Verification items for this drawing (mm, ordinates from the low corner). A direction names the side the tool comes from. Round coordinates to 2 decimals unless told otherwise and drop trailing zeros. Order: outer loops, then holes, each group sorted by start corner. A loop starts at its lowest first (then second) coordinate and runs counter-clockwise, first axis right, second up. Notation, with made-up numbers: (61, 87) -> (116, 87) arc R11 ccw to (116, 107) -> close; hole circle Ø5 at (88.5, 22.25). An arc over 180 degrees is marked (long way). Return JSON: item names as keys, results as strings. Group by question number.
Item 1: Sectioned sample at B-B on x = 114.3. Record the cut outline in (y, z).
Item 2: Access from +Z, -Z, +X, -X, +Y, -Y to the whole of each face (thin tool, end or side, straight path). Record for the marked faces 1, 2, 3, 4 and 5.
Item 3: Scan lines: probe 1 along Z at (x, y) = (31, 31.5); probe 2 along X at (y, z) = (19.05, 36); probe 3 along Y at (x, z) = (114.3, 28). Record each from-to range of solid material in increasing order. Write a range as from..to.
Item 4: Depth check by flat-ended pin: pin 1 Ø2 at (y, z) = (10.5, 32) entering from -X; pin 2 Ø6 at (y, z) = (29.5, 14) entering from -X; pin 3 Ø14.5 at (x, y) = (12.7, 19.05) entering from -Z; pin 4 Ø6 at (x, z) = (57, 23) entering from -Y. Enter the tip coordinate at first touch or a pass-through.
Item 5: Sectioned sample at A-A on z = 27. Record the cut outline in (x, y) (3 decimals), plus the area to 3 significant figures.
Item 6: Sectioned sample at D-D on x = 15.5. Record the cut outline in (y, z), plus the area to 3 significant figures.
Item 7: Sectioned sample at C-C on y = 10.5. Give the number of separate pieces and of enclosed holes in the cut face, plus the area to 3 significant figures.
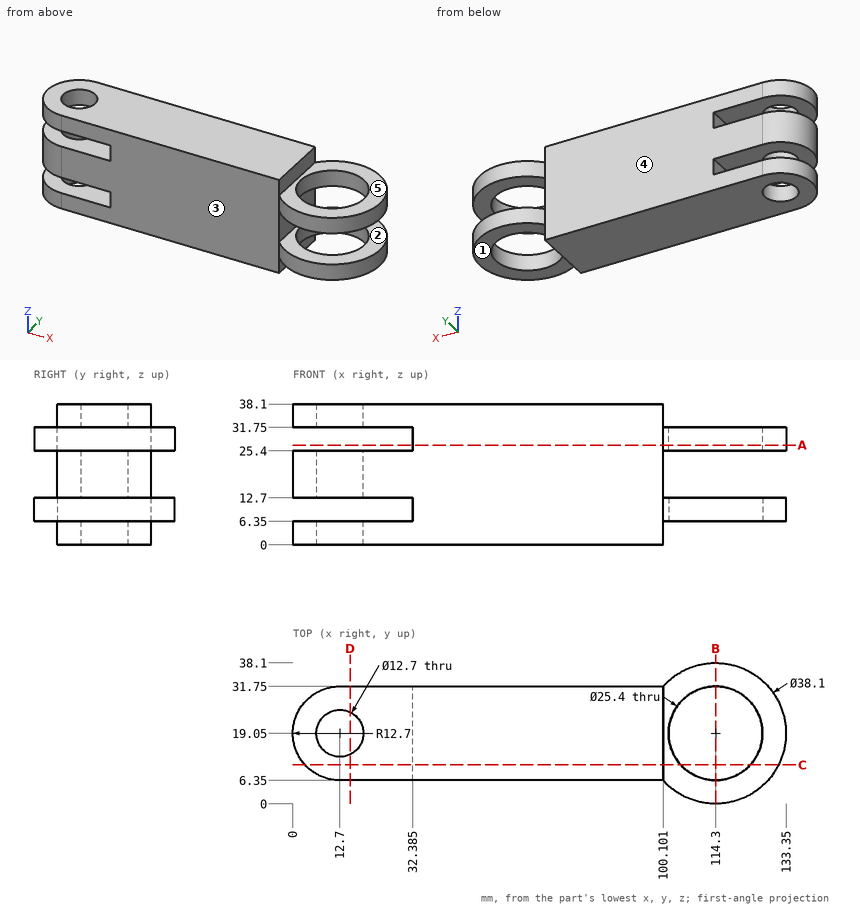
Recorded:
{
 "1": {"outline": "(0, 6.35) -> (6.35, 6.35) -> (6.35, 12.7) -> (0, 12.7) -> close; (0, 25.4) -> (6.35, 25.4) -> (6.35, 31.75) -> (0, 31.75) -> close; (31.75, 6.35) -> (38.1, 6.35) -> (38.1, 12.7) -> (31.75, 12.7) -> close; (31.75, 25.4) -> (38.1, 25.4) -> (38.1, 31.75) -> (31.75, 31.75) -> close"},
 "2": {"face 1": "-Z, +X, +Y, -Y", "face 2": "+X, +Y, -Y", "face 3": "+Z, -Z, -X, -Y", "face 4": "+Z, -Z, -X, +Y", "face 5": "+Z, +X, +Y, -Y"},
 "3": {"probe 1": "0..6.35, 12.7..25.4, 31.75..38.1", "probe 2": "0..6.35, 19.05..100.1", "probe 3": "0..6.35, 31.75..38.1"},
 "4": {"pin 1": "x = 2.49", "pin 2": "x = 2.41", "pin 3": "z = 0", "pin 4": "y = 6.35"},
 "5": {"outline": "(32.385, 6.35) -> (100.101, 6.35) arc R19.05 ccw (long way) to (100.101, 31.75) -> (32.385, 31.75) -> close; hole circle Ø25.4 at (114.3, 19.05)", "area": "2,270 mm²"},
 "6": {"outline": "(6.35, 0) -> (13.35, 0) -> (13.35, 6.35) -> (6.35, 6.35) -> close; (6.35, 12.7) -> (13.35, 12.7) -> (13.35, 25.4) -> (6.35, 25.4) -> close; (6.35, 31.75) -> (13.35, 31.75) -> (13.35, 38.1) -> (6.35, 38.1) -> close; (24.75, 0) -> (31.75, 0) -> (31.75, 6.35) -> (24.75, 6.35) -> close; (24.75, 12.7) -> (31.75, 12.7) -> (31.75, 25.4) -> (24.75, 25.4) -> close; (24.75, 31.75) -> (31.75, 31.75) -> (31.75, 38.1) -> (24.75, 38.1) -> close", "area": "356 mm²"},
 "7": {"separate pieces": "3", "enclosed holes": "0", "area": "3,480 mm²"}
}
